from build123d import *

# Parameters (mm, degrees)
SKETCH1_W           = 57
SKETCH1_H           = 67
BOSS_EXTRUDE1_DEPTH = 20
SKETCH2_R           = 1.7
CUT_EXTRUDE1_DEPTH  = 20
SKETCH3_W           = 28
SKETCH3_H           = 20
BOSS_EXTRUDE2_DEPTH = 25


with BuildPart() as part:
    # Sketch1 → Boss-Extrude1 (new body)
    with BuildSketch(Plane(origin=(0, 0, 0), x_dir=(1, 0, 0), z_dir=(0, 1, 0))):
        Rectangle(SKETCH1_W, SKETCH1_H)
    extrude(amount=BOSS_EXTRUDE1_DEPTH)

    # Sketch2 → Cut-Extrude1 (cut)
    with BuildSketch(Plane(origin=(0, 20, 0), x_dir=(1, 0, 0), z_dir=(0, 1, 0))):
        with Locations(Location((-24.5, 27.5, 0), (0, 0, 270))):
            Circle(SKETCH2_R)
        with Locations(Location((23.5, 27.5, 0), (0, 0, 270))):
            Circle(SKETCH2_R)
        with Locations(Location((23.5, -20.5, 0), (0, 0, 270))):
            Circle(SKETCH2_R)
    extrude(amount=-CUT_EXTRUDE1_DEPTH, mode=Mode.SUBTRACT)

    # Sketch3 → Boss-Extrude2 (add)
    with BuildSketch(Plane(origin=(0, 0, -33.5), x_dir=(-1, 0, 0), z_dir=(0, 0, -1))):
        with Locations((14.5, 10)):
            Rectangle(SKETCH3_W, SKETCH3_H)
    extrude(amount=BOSS_EXTRUDE2_DEPTH)


solid = part.part
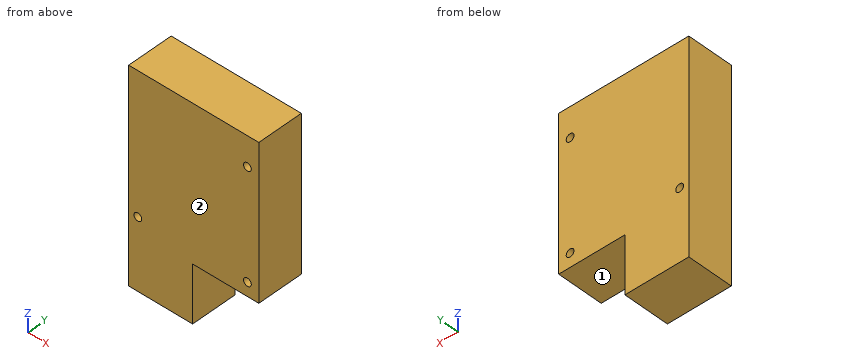
Input: part model. Units: mm. Frame: model coordinates. Face numbers are marked on the shaded views. A direction names the side the tool comes from. Give positions to 0.01 mm unless a question says otherwise; leave off trailing zeros. Write each loop counter-clockwise with the first axis right and the second up, starting at its lowest first coordinate (ties: lowest second). Pieces come first, ordered by that corner, then holes. Notation, with made-up numbers: (78.5, 31) -> (118.5, 31) arc R22 cw to (118.5, 45) -> close; hole circle Ø1 at (49, 56). An arc over 180 degrees is marked (long way). Use one line per item in the form item = value. Start each with the question number.
1) Pin query (flat end, axial travel): pin 1 (12 mm diameter, centred on y = 17, z = -42, fed in from +X); pin 2 (2 mm diameter, centred on x = 9, y = 6, fed in from -Z); pin 3 (2 mm diameter, centred on x = 11, z = -24.5, fed in from -Y). Return the tip coordinate at first contact, or that it passes through.
2) Ray query, probe 1 along X at (y, z) = (14, -27.5); probe 2 along Z at (x, y) = (22, 7.5); probe 3 along X at (y, z) = (9.5, -26). Return the intervals inside material, ascending. Write a range as from..to.
3) Section query A-A on y = 14. Return the cut outline in (x, z), then the cut area to 3 significant figures.
4) Section query C-C on x = 23.5. Return the cut outline in (y, z).
5) Section query D-D on x = -24.5. Return the cut outline in (y, z), then the cut area to 3 significant figures.
6) Set-up query: the marked faces 1 and 2. Return all of +Z, -Z, +X, -X, +Y, -Y with unobstructed straight access to the full face (end or side cutting, diameter ignored); none if empty.
7) Section query B-B on z = 20.5. Return the cut outline in (x, y).
Outcome:
q1.pin_1 = -0.5
q1.pin_2 = -33.5
q1.pin_3 = 0
q2.probe_1 = -28.5..-26.2, -22.8..21.8, 25.2..28.5
q2.probe_2 = -33.5..-28.3, -26.7..19.7, 21.3..33.5
q2.probe_3 = -28.5..-25.3, -23.7..22.7, 24.3..28.5
q3.outline = (-28.5, -58.5) -> (-0.5, -58.5) -> (-0.5, -33.5) -> (28.5, -33.5) -> (28.5, 33.5) -> (-28.5, 33.5) -> close; hole circle Ø3.4 at (-24.5, -27.5); hole circle Ø3.4 at (23.5, -27.5); hole circle Ø3.4 at (23.5, 20.5)
q3.area = 4,490 mm^2
q4.outline = (0, -33.5) -> (20, -33.5) -> (20, -29.2) -> (0, -29.2) -> close; (0, -25.8) -> (20, -25.8) -> (20, 18.8) -> (0, 18.8) -> close; (0, 22.2) -> (20, 22.2) -> (20, 33.5) -> (0, 33.5) -> close
q5.outline = (0, -58.5) -> (20, -58.5) -> (20, -29.2) -> (0, -29.2) -> close; (0, -25.8) -> (20, -25.8) -> (20, 33.5) -> (0, 33.5) -> close
q5.area = 1,770 mm^2
q6.face_1 = -Z, +X, +Y, -Y
q6.face_2 = +Z, -Z, +X, -X, -Y
q7.outline = (-28.5, 0) -> (21.8, 0) -> (21.8, 20) -> (-28.5, 20) -> close; (25.2, 0) -> (28.5, 0) -> (28.5, 20) -> (25.2, 20) -> close
